Check sheet for the drawn part. Datum: minimum x, y, z corner. Units: mm. A direction names the side the tool comes from. Give positions to 0.01 mm unless a question says otherwise; leave off trailing zeros. Write each loop counter-clockwise with the first axis right and the second up, starting at its lowest first coordinate (ties: lowest second). Pieces come first, ordered by that corner, then holes. Notation, with made-up numbers: M -30,-28 L 0,-28 A15 cw 0,-17 Z; hole C 35.25,57.25 d11. An arc over 180 degrees is marked long. Write item = value, one per line.
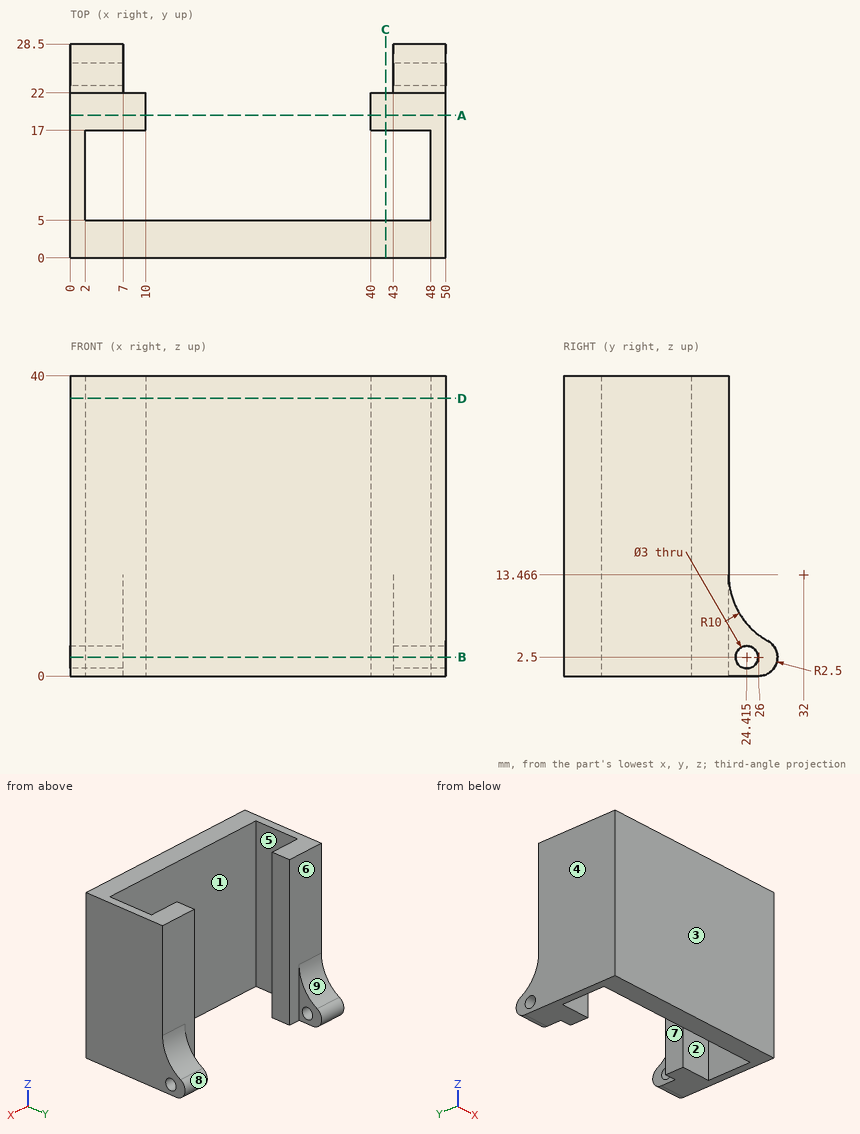
1) Material ranges on probe 1 along Y at (x, z) = (4, 2.5) (1 decimal); probe 2 along Y at (x, z) = (5.5, 16.5); probe 3 along X at (y, z) = (6, 23.5), recorded low to high. Write a range as from..to.
From the geometry:
probe_1 = 0..5, 17..22.9, 25.9..28.5
probe_2 = 0..5, 17..22
probe_3 = 0..2, 48..50
2) Cross-section at D-D on z = 37. Record the boundary of the cut face in (x, y).
From the geometry:
outline = M 0,0 L 50,0 L 50,22 L 40,22 L 40,17 L 48,17 L 48,5 L 2,5 L 2,17 L 10,17 L 10,22 L 0,22 Z
3) Tool access check on the marked faces 5, 6, 7, 8 and 9. Record the directions out of +Z, -Z, +X, -X, +Y, -Y that give a thin tool (end or side, any length) a straight path to the whole face; none if there is none.
From the geometry:
face_5 = +Z, -Z
face_6 = +Z, +Y
face_7 = +Z, -Z, +Y
face_8 = +X, -X, +Y
face_9 = +Z, +X, -X, +Y
4) Depth check by flat-ended pin: P1, Ø5, axis at y = 24.41, z = 2.5, coming from the -X side; P2, Ø3, axis at x = 33.5, z = 31, coming from the +Y side; P3, Ø3, axis at x = 7.5, z = 14.5, coming from the +Y side. Enter the tip coordinate at first touch or a pass-through.
From the geometry:
P1 = 0
P2 = 5
P3 = 22.01
5) Draft check along Y on the marked faces 1, 2, 3 and 4. Enter one of: +Y half, -Y half, draft (parallel to the pull), parting line (faces both ways), or undercut.
From the geometry:
face_1 = undercut
face_2 = undercut
face_3 = -Y half
face_4 = draft
6) Cross-section at A-A on y = 19. Record the boundary of the cut face in (x, z), plus the area to 3 significant figures.
From the geometry:
outline = M 0,0 L 10,0 L 10,40 L 0,40 Z; M 40,0 L 50,0 L 50,40 L 40,40 Z
area = 800 mm^2
7) Cross-section at C-C on x = 42. Record the boundary of the cut face in (y, z).
From the geometry:
outline = M 0,0 L 5,0 L 5,40 L 0,40 Z; M 17,0 L 22,0 L 22,40 L 17,40 Z
8) Cross-section at B-B on z = 2.5. Record the boundary of the cut face in (x, y) (1 decimal), plus the area to 3 significant figures.
From the geometry:
outline = M 0,0 L 50,0 L 50,22.9 L 43,22.9 L 43,22 L 40,22 L 40,17 L 48,17 L 48,5 L 2,5 L 2,17 L 10,17 L 10,22 L 7,22 L 7,22.9 L 0,22.9 Z; M 0,25.9 L 7,25.9 L 7,28.5 L 0,28.5 Z; M 43,25.9 L 50,25.9 L 50,28.5 L 43,28.5 Z
area = 447 mm^2
